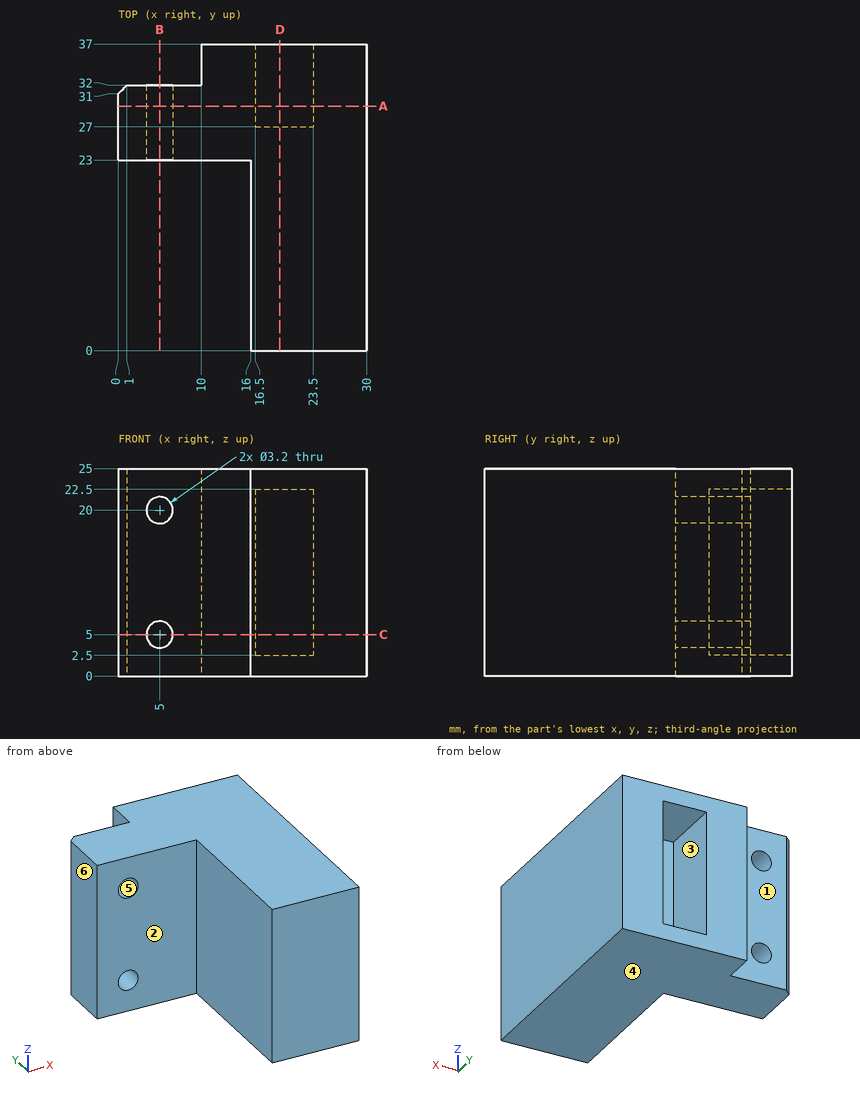
Drawing for the job (mm, zero at the part's lowest x, y, z). A direction names the side the tool comes from. Round coordinates to 2 decimals unless told otherwise and drop trailing zeros. Order: outer loops, then holes, each group sorted by start corner. A loop starts at its lowest first (then second) coordinate and runs counter-clockwise, first axis right, second up.
Item 1: Tool access for the marked faces 1, 2 and 3: list every direction of +Z, -Z, +X, -X, +Y, -Y with a clear straight run to the whole face (end or side of a thin tool).
Item 2: Saw through at C-C on z = 5. Write the cut outline in (x, y), then the cut area to 3 significant figures.
Item 3: Saw through at D-D on x = 19.5. Write the cut outline in (y, z), then the cut area to 3 significant figures.
Item 4: Pin check, flat tips, straight feed: pin 1 (1 mm diameter, centred on x = 12.5, z = 15, fed in from -Y); pin 2 (10 mm diameter, centred on x = 3.5, z = 20, fed in from +Y); pin 3 (8 mm diameter, centred on x = 22.5, y = 15.5, fed in from -Z); pin 4 (5.5 mm diameter, centred on y = 34, z = 8, fed in from -X). Stop position of each tip, or through.
Item 5: Saw through at A-A on y = 29.5. Write the cut outline in (x, z).
Item 6: Saw through at B-B on x = 5. Write the cut outline in (y, z), then the cut area to 3 significant figures.
Item 7: Probe line 1 along Z through (x, y) = (5, 31); line 2 along X through (y, z) = (27.5, 20); line 3 along X through (y, z) = (32.5, 17.25). List the from-to ranges inside material, lowest first.
Item 8: Mould opens along Z. For the marked faces 4, 5 and 6 say: pulls with the +Z half, pulls with the -Z half, needs draft (parallel to the pull), parting line crosses it, or undercut.
Reported:
1. face 1: +Z, -Z, -X, +Y
1. face 2: +Z, -Z, -X, -Y
1. face 3: +Y
2. outline: (0, 23) - (3.4, 23) - (3.4, 32) - (1, 32) - (0, 31) - close; (6.6, 23) - (16, 23) - (16, 0) - (30, 0) - (30, 37) - (23.5, 37) - (23.5, 27) - (16.5, 27) - (16.5, 37) - (10, 37) - (10, 32) - (6.6, 32) - close
2. area: 593 mm2
3. outline: (0, 0) - (37, 0) - (37, 2.5) - (27, 2.5) - (27, 22.5) - (37, 22.5) - (37, 25) - (0, 25) - close
3. area: 725 mm2
4. pin 1: stops at y = 23
4. pin 2: stops at y = 32
4. pin 3: stops at z = 0
4. pin 4: stops at x = 0.25
5. outline: (0, 0) - (30, 0) - (30, 25) - (0, 25) - close; hole circle Ø3.2 at (5, 5); hole circle Ø3.2 at (5, 20); hole (16.5, 2.5) - (23.5, 2.5) - (23.5, 22.5) - (16.5, 22.5) - close
6. outline: (23, 0) - (32, 0) - (32, 3.4) - (23, 3.4) - close; (23, 6.6) - (32, 6.6) - (32, 18.4) - (23, 18.4) - close; (23, 21.6) - (32, 21.6) - (32, 25) - (23, 25) - close
6. area: 167 mm2
7. line 1: z = 0 to 3.4, 6.6 to 18.4, 21.6 to 25
7. line 2: x = 0 to 3.4, 6.6 to 16.5, 23.5 to 30
7. line 3: x = 10 to 16.5, 23.5 to 30
8. face 4: pulls with the -Z half
8. face 5: undercut
8. face 6: needs draft
